Design review of the part built by this model. Coordinates are the model's own, in mm. Round coordinates to 2 decimals unless told otherwise and drop trailing zeros. Write each loop counter-clockwise with the first axis right and the second up, starting at its lowest first coordinate (ties: lowest second). Pieces come first, ordered by that corner, then holes. Notation, with made-up numbers: (33, 86.5) -> (41, 86.5) arc R32 ccw to (41, 117.5) -> close; hole circle Ø5 at (-25, 7.25). An arc over 180 degrees is marked (long way). Write item = value, one per line. Start each with the question number.
Item 1: Add section B-B, the plane y = 0. State the section outline as (x, z) points.
Item 2: To check wall thickness, follow L1, parallel to X at y = 0, z = 71; L2, parallel to Y at x = -7.5, z = 11.5. State the ranges of each line that lie inside material, in increasing order.
Item 3: Add section A-A, the plane x = 0. State the section outline as (y, z) points.
Item 4: Mouldability with a two-part tool opening along Y and no side actions: class faces 1 (the cylindrical face through (10, 3.2, 49.3)), 2 (the cylindrical face through (-11.99, 0.53, 49.3)), 3 (the flat face through (0, -11, 100)) as released by +Y, released by -Y, zero draft, split by the parting line, or undercut.
Item 5: Add section C-C, the plane z = 54. State the section outline as (x, y) points, then the cut area to 3 significant figures.
Item 6: For pin 1 Ø4 at (y, z) = (4.5, 49) entering from +X; pin 2 Ø1.2 at (x, z) = (-11.5, 1.5) entering from -Y; pin 3 Ø0.8 at (x, y) = (11.5, -0.5) entering from -Z, all flat-tipped, find the tip position at first contact; note any pin that passes through.
from build123d import *

# Parameters (mm, degrees)
F0_R     = 12
F0_R_2   = 10.5
F1_DEPTH = 100
F2_W     = 2
F2_H     = 2
F3_DEPTH = 15.56


with BuildPart() as f1:
    # F0 (on Top) → F1 (new body)
    with BuildSketch(Plane.XY):
        Circle(F0_R)
        Circle(F0_R_2, mode=Mode.SUBTRACT)
    extrude(amount=F1_DEPTH)

    # F2 (on Right) → F3 (cut, symmetric)
    with BuildSketch(Plane.YZ):
        with Locations((0, 1)):
            Rectangle(F2_W, F2_H)
    extrude(amount=F3_DEPTH, both=True, mode=Mode.SUBTRACT)


solid = f1.part
Result set:
q1.outline = (-12, 2) -> (-10.5, 2) -> (-10.5, 100) -> (-12, 100) -> close; (10.5, 2) -> (12, 2) -> (12, 100) -> (10.5, 100) -> close
q2.L1 = -12 to -10.5, 10.5 to 12
q2.L2 = -9.37 to -7.35, 7.35 to 9.37
q3.outline = (-12, 0) -> (-10.5, 0) -> (-10.5, 100) -> (-12, 100) -> close; (10.5, 0) -> (12, 0) -> (12, 100) -> (10.5, 100) -> close
q4.face_1 = undercut
q4.face_2 = split by the parting line
q4.face_3 = zero draft
q5.outline = circle Ø24 at (0, 0); hole circle Ø21 at (0, 0)
q5.area = 106 mm²
q6.pin_1 = 11.74
q6.pin_2 = -5.02
q6.pin_3 = 2
